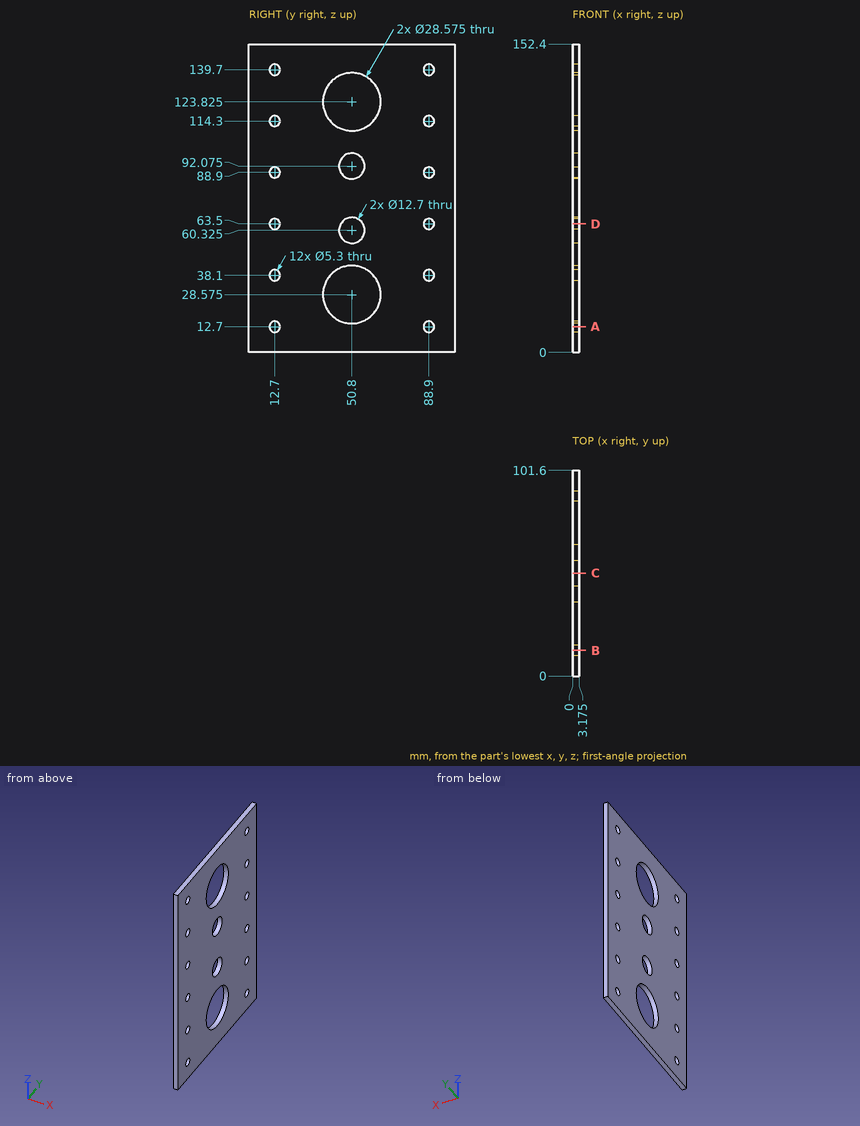
Could you check a few things on this drawing? It's one solid part, dimensions in mm from its lowest x, y, z. Coordinates: 2 decimals unless noted, no trailing zeros. Order: outer loops, then holes, each group sorted by start corner. A loop starts at its lowest first (then second) coordinate and runs counter-clockwise, first axis right, second up.
1) Will this pin go through, and if not, where does the flat tip stop? pin 1 (8.5 mm diameter, centred on y = 12.7, z = 139.7, fed in from +X) (3 decimals).
2) Imagine slicing it at D-D on z = 63.5. List the corners of the cut face in (x, y) for me (3 decimals), and give its area (3 significant figures).
3) I need wall thicknesses on line 1 (Z direction, x = 1.65, y = 50.8) (1 decimal); line 2 (Z direction, x = 1.5, y = 40); line 3 (Z direction, x = 2.9, y = 62). Which ranges of each line are inside material? Lowest first, please.
4) Imagine slicing it at C-C on y = 50.8. List the corners of the cut face in (x, z) for me (1 decimal).
5) Imagine slicing it at A-A on z = 12.7. List the corners of the cut face in (x, y) for me (3 decimals), and give its area (3 significant figures).
6) Imagine slicing it at B-B on y = 12.7. List the corners of the cut face in (x, z) for me (3 decimals).
Response values:
1. pin 1: stops at x = 3.175
2. outline: (0, 0) - (3.175, 0) - (3.175, 10.05) - (0, 10.05) - close; (0, 15.35) - (3.175, 15.35) - (3.175, 45.301) - (0, 45.301) - close; (0, 56.299) - (3.175, 56.299) - (3.175, 86.25) - (0, 86.25) - close; (0, 91.55) - (3.175, 91.55) - (3.175, 101.6) - (0, 101.6) - close
2. area: 254 mm2
3. line 1: z = 0 to 14.3, 42.9 to 54, 66.7 to 85.7, 98.4 to 109.5, 138.1 to 152.4
3. line 2: z = 0 to 19.22, 37.93 to 114.47, 133.18 to 152.4
3. line 3: z = 0 to 19.7, 37.45 to 114.95, 132.7 to 152.4
4. outline: (0, 0) - (3.2, 0) - (3.2, 14.3) - (0, 14.3) - close; (0, 42.9) - (3.2, 42.9) - (3.2, 54) - (0, 54) - close; (0, 66.7) - (3.2, 66.7) - (3.2, 85.7) - (0, 85.7) - close; (0, 98.4) - (3.2, 98.4) - (3.2, 109.5) - (0, 109.5) - close; (0, 138.1) - (3.2, 138.1) - (3.2, 152.4) - (0, 152.4) - close
5. outline: (0, 0) - (3.175, 0) - (3.175, 10.05) - (0, 10.05) - close; (0, 15.35) - (3.175, 15.35) - (3.175, 86.25) - (0, 86.25) - close; (0, 91.55) - (3.175, 91.55) - (3.175, 101.6) - (0, 101.6) - close
5. area: 289 mm2
6. outline: (0, 0) - (3.175, 0) - (3.175, 10.05) - (0, 10.05) - close; (0, 15.35) - (3.175, 15.35) - (3.175, 35.45) - (0, 35.45) - close; (0, 40.75) - (3.175, 40.75) - (3.175, 60.85) - (0, 60.85) - close; (0, 66.15) - (3.175, 66.15) - (3.175, 86.25) - (0, 86.25) - close; (0, 91.55) - (3.175, 91.55) - (3.175, 111.65) - (0, 111.65) - close; (0, 116.95) - (3.175, 116.95) - (3.175, 137.05) - (0, 137.05) - close; (0, 142.35) - (3.175, 142.35) - (3.175, 152.4) - (0, 152.4) - close
